from build123d import *

# Parameters (mm, degrees)
SKETCH1_W            = 164
SKETCH1_H            = 264
BOSS_EXTRUDE1_DEPTH  = 4
CUT_EXTRUDE3_DEPTH   = 10
CUT_EXTRUDE4_DEPTH   = 10
LPATTERN1_COUNT      = 3
LPATTERN1_PITCH      = 10
LPATTERN1_COUNT_DIR2 = 2
LPATTERN1_PITCH_DIR2 = 50
CUT_EXTRUDE5_DEPTH   = 10
SKETCH5_W            = 4.319122357
SKETCH5_H            = 26.937684175
SKETCH5_H_2          = 25.730682063
BOSS_EXTRUDE2_DEPTH  = 4
FILLET3_R            = 5
FILLET4_R            = 5
FILLET5_R            = 4.5
FILLET6_R            = 4.5
FILLET7_R            = 4.75
FILLET8_R            = 4.75
FILLET9_R            = 4.5
FILLET10_R           = 4.5


with BuildPart() as part:
    # Sketch1 → Boss-Extrude1 (new body)
    with BuildSketch(Plane.XY):
        with Locations((12.541176471, -29.098039216)):
            Rectangle(SKETCH1_W, SKETCH1_H)
    extrude(amount=BOSS_EXTRUDE1_DEPTH)

    # Sketch2 → Cut-Extrude3 (cut)
    with BuildSketch(Plane.XY.offset(4)):
        with BuildLine():
            ThreePointArc((-19.196819428, 52.401960784), (13.041176471, 20.163964886), (45.279172369, 52.401960784))
            ThreePointArc((45.279172369, 52.401960784), (40.932647519, 56.748485634), (36.58612267, 52.401960784))
            ThreePointArc((36.58612267, 52.401960784), (13.041176471, 28.857014585), (-10.503769729, 52.401960784))
            ThreePointArc((-10.503769729, 52.401960784), (-14.850294578, 56.748485634), (-19.196819428, 52.401960784))
        make_face()
        with BuildLine():
            ThreePointArc((33.426584493, 52.401960784), (13.041176471, 72.787368807), (-7.344231552, 52.401960784))
            ThreePointArc((-7.344231552, 52.401960784), (-2.891363068, 47.949092301), (1.561505415, 52.401960784))
            ThreePointArc((1.561505415, 52.401960784), (13.041176471, 63.88163184), (24.520847526, 52.401960784))
            ThreePointArc((24.520847526, 52.401960784), (28.97371601, 47.949092301), (33.426584493, 52.401960784))
        make_face()
        with BuildLine():
            ThreePointArc((42.181568033, 67.499048907), (12.784631297, 85.219923468), (-16.331673874, 67.04163813))
            ThreePointArc((-16.331673874, 67.04163813), (-14.055015917, 60.240559274), (-7.253937061, 62.517217231))
            ThreePointArc((-7.253937061, 62.517217231), (12.863917084, 75.077467953), (33.17567306, 62.833264313))
            ThreePointArc((33.17567306, 62.833264313), (40.011512844, 60.663209124), (42.181568033, 67.499048907))
        make_face()
        with BuildLine():
            ThreePointArc((-3.609454357, 38.710399181), (12.244809645, 30.859719351), (28.635450382, 37.518379654))
            ThreePointArc((28.635450382, 37.518379654), (28.481389363, 44.125242049), (21.874526968, 43.97118103))
            ThreePointArc((21.874526968, 43.97118103), (12.590075808, 40.199393986), (3.609454357, 44.646398506))
            ThreePointArc((3.609454357, 44.646398506), (-2.967999663, 45.2878532), (-3.609454357, 38.710399181))
        make_face()
    extrude(amount=-CUT_EXTRUDE3_DEPTH, mode=Mode.SUBTRACT)

    # Sketch3 → Cut-Extrude4 (cut)
    with BuildSketch(Plane.XY.offset(4)):
        with BuildLine():
            Line((76.541176471, -57.098039216), (46.541176471, -57.098039216))
            ThreePointArc((46.541176471, -57.098039216), (44.541176471, -55.098039216), (46.541176471, -53.098039216))
            Line((46.541176471, -53.098039216), (76.541176471, -53.098039216))
            ThreePointArc((76.541176471, -53.098039216), (78.541176471, -55.098039216), (76.541176471, -57.098039216))
        make_face()
    cut_extrude4 = extrude(amount=-CUT_EXTRUDE4_DEPTH, mode=Mode.SUBTRACT)

    # LPattern1: Cut-Extrude4 3 × 2
    with Locations(*[(-j * LPATTERN1_PITCH_DIR2, -i * LPATTERN1_PITCH, 0) for i in range(LPATTERN1_COUNT) for j in range(LPATTERN1_COUNT_DIR2) if (i, j) != (0, 0)]):
        add(cut_extrude4, mode=Mode.SUBTRACT)

    # Sketch4 → Cut-Extrude5 (cut)
    with BuildSketch(Plane.XY.offset(4)):
        with BuildLine():
            Line((7.541176471, -143.598039216), (17.541176471, -143.598039216))
            ThreePointArc((17.541176471, -143.598039216), (20.041176471, -146.098039216), (17.541176471, -148.598039216))
            Line((17.541176471, -148.598039216), (7.541176471, -148.598039216))
            ThreePointArc((7.541176471, -148.598039216), (5.041176471, -146.098039216), (7.541176471, -143.598039216))
        make_face()
    extrude(amount=-CUT_EXTRUDE5_DEPTH, mode=Mode.SUBTRACT)

    # Sketch5 → Boss-Extrude2 (add)
    with BuildSketch(Plane.XY.offset(4)):
        with Locations((13.038358708, 73.546081582)):
            Rectangle(SKETCH5_W, SKETCH5_H)
        with Locations((13.038358708, 29.708086806)):
            Rectangle(SKETCH5_W, SKETCH5_H_2)
    extrude(amount=-BOSS_EXTRUDE2_DEPTH)

    # Fillet3
    fillet3_edges = [part.edges().sort_by_distance(p)[0] for p in [
        (15.197919886, 74.975363365, 2),
        (15.197919886, 85.149982831, 2),
    ]]
    fillet(fillet3_edges, radius=FILLET3_R)

    # Fillet4
    fillet4_edges = [part.edges().sort_by_distance(p)[0] for p in [
        (10.878797529, 74.974824217, 2),
        (10.878797529, 85.149611196, 2),
    ]]
    fillet(fillet4_edges, radius=FILLET4_R)

    # Fillet5
    # the kernel refuses this fillet: 4.5 mm, written as the material it adds along each edge
    with BuildSketch(Plane(origin=(10.878797529, 63.676133253, 0), x_dir=(-0.952400444463688, -0.3048497882324502, 0), z_dir=(0, 0, 1))) as fillet5_piece_1:
        with BuildLine():
            CenterArc((3.294924666, -4.467486403), FILLET5_R, 96.891689821, 65.359183141)
            Line((-0.990877334, -3.095662356), (0, 0))
            ThreePointArc((0, 0), (1.377478425, -0.082943423), (2.75495685, 0))
        make_face()
    extrude(amount=4)
    with BuildSketch(Plane(origin=(10.878797529, 72.672357366, 0), x_dir=(0, -1, 0), z_dir=(0, 0, 1))) as fillet5_piece_2:
        with BuildLine():
            CenterArc((5.849616613, -4.5), FILLET5_R, 90, 114.796867003)
            ThreePointArc((1.764514753, -6.387310996), (0.620984955, -3.265832826), (0, 0))
            Line((0, 0), (5.849616613, 0))
        make_face()
    extrude(amount=4)

    # Fillet6
    # the kernel refuses this fillet: 4.5 mm, written as the material it adds along each edge
    with BuildSketch(Plane(origin=(15.197919886, 72.672957753, 0), x_dir=(0.963984906204346, -0.2659569525509686, 0), z_dir=(0, 0, 1))) as fillet6_piece_1:
        with BuildLine():
            CenterArc((5.893145872, -4.440206052), FILLET6_R, 80.649344531, 114.774478291)
            Line((1.555213794, -5.637012339), (0, 0))
            ThreePointArc((0, 0), (3.312144479, 0.270872005), (6.624288959, 0))
        make_face()
    extrude(amount=4)
    with BuildSketch(Plane(origin=(15.197919886, 63.677212683, 0), x_dir=(0.9525356739175572, -0.30442698617965064, 0), z_dir=(0, 0, 1))) as fillet6_piece_2:
        with BuildLine():
            CenterArc((3.296449531, 4.467456192), FILLET6_R, 197.723693353, 65.381411924)
            Line((-0.989961002, 3.097534754), (0, 0))
            ThreePointArc((0, 0), (1.378115911, 0.083020491), (2.756231822, 0))
        make_face()
    extrude(amount=4)

    # Fillet7
    # the kernel refuses this fillet: 4.75 mm, written as the material it adds along each edge
    with BuildSketch(Plane(origin=(15.197919886, 30.953165389, 0), x_dir=(0, 1, 0), z_dir=(0, 0, 1))) as fillet7_piece_1:
        with BuildLine():
            CenterArc((6.126567217, -4.75), FILLET7_R, 90, 114.26424477)
            ThreePointArc((1.796182676, -6.701991222), (0.626677135, -3.423736603), (0, 0))
            Line((0, 0), (6.126567217, 0))
        make_face()
    extrude(amount=4)
    with BuildSketch(Plane(origin=(15.197919886, 40.383034621, 0), x_dir=(0.9557846908185708, 0.2940673813887714, 0), z_dir=(0, 0, 1))) as fillet7_piece_2:
        with BuildLine():
            CenterArc((3.51897249, -4.715313748), FILLET7_R, 96.928419065, 65.969959025)
            Line((-1.021004791, -3.318493687), (0, 0))
            ThreePointArc((0, 0), (1.472991805, -0.08916851), (2.94598361, 0))
        make_face()
    extrude(amount=4)

    # Fillet8
    # the kernel refuses this fillet: 4.75 mm, written as the material it adds along each edge
    with BuildSketch(Plane(origin=(10.878797529, 40.384047255, 0), x_dir=(0, -1, 0), z_dir=(0, 0, 1))) as fillet8_piece_1:
        with BuildLine():
            CenterArc((3.470508434, -4.75), FILLET8_R, 90, 65.949113414)
            ThreePointArc((-0.867114896, -2.814147772), (-0.348416422, -1.433308135), (0, 0))
            Line((0, 0), (3.470508434, 0))
        make_face()
    extrude(amount=4)
    with BuildSketch(Plane(origin=(10.878797529, 30.953732806, 0), x_dir=(-0.9658301221176608, 0.2591759541511984, 0), z_dir=(0, 0, 1))) as fillet8_piece_2:
        with BuildLine():
            CenterArc((6.176063632, -4.688044059), FILLET8_R, 80.735851864, 114.285319943)
            Line((1.588370552, -5.919129841), (0, 0))
            ThreePointArc((0, 0), (3.470374234, 0.281175054), (6.940748468, 0))
        make_face()
    extrude(amount=4)

    # Fillet9
    # the kernel refuses this fillet: 4.5 mm, written as the material it adds along each edge
    with BuildSketch(Plane(origin=(10.878797529, 20.23656794, 0), x_dir=(0, 1, 0), z_dir=(0, 0, 1))) as fillet9_piece_1:
        with BuildLine():
            CenterArc((5.239399394, 4.5), FILLET9_R, 166.10226732, 103.89773268)
            ThreePointArc((0.871132452, 5.58085333), (0.313102845, 2.809542348), (0, 0))
            Line((0, 0), (5.239399394, 0))
        make_face()
    extrude(amount=4)
    with BuildSketch(Plane(origin=(10.878797529, 28.956521807, 0), x_dir=(-0.9862681446857605, 0.16515189002281502, 0), z_dir=(0, 0, 1))) as fillet9_piece_2:
        with BuildLine():
            CenterArc((3.811181811, 4.487703929), FILLET9_R, 189.50605818, 76.257380527)
            Line((-0.62702484, 3.744520424), (0, 0))
            ThreePointArc((0, 0), (1.739373093, 0.064335629), (3.478746186, 0))
        make_face()
    extrude(amount=4)

    # Fillet10
    # the kernel refuses this fillet: 4.5 mm, written as the material it adds along each edge
    with BuildSketch(Plane(origin=(15.197919886, 20.236189577, 0), x_dir=(0.9880653050237032, 0.15403555761062557, 0), z_dir=(0, 0, 1))) as fillet10_piece_1:
        with BuildLine():
            CenterArc((5.253191268, 4.482705444), FILLET10_R, 171.139133949, 103.885741164)
            Line((0.806897395, 5.175865453), (0, 0))
            ThreePointArc((0, 0), (2.823669163, -0.123898184), (5.647338326, 0))
        make_face()
    extrude(amount=4)
    with BuildSketch(Plane(origin=(15.197919886, 28.956002724, 0), x_dir=(0.9863050503076972, 0.16493134249599425, 0), z_dir=(0, 0, 1))) as fillet10_piece_2:
        with BuildLine():
            CenterArc((3.812043631, -4.48769836), FILLET10_R, 94.237521054, 76.269232907)
            Line((-0.626329096, -3.745507319), (0, 0))
            ThreePointArc((0, 0), (1.739766416, -0.064364768), (3.479532832, 0))
        make_face()
    extrude(amount=4)


solid = part.part
Here's how the part is built. I have some questions about the finished solid (model axes, mm). A direction names the side the tool comes from. Give positions to 0.01 mm unless a question says otherwise; leave off trailing zeros. Loops run counter-clockwise (first coordinate to the right, second up) from the corner with the lowest first, then second, coordinate; pieces in that order, holes last. Notation, with made-up numbers: (57, 19) -> (116, 19) arc R19 ccw to (116, 29) -> close; hole circle Ø11 at (72, -37.75). An arc over 180 degrees is marked (long way). Answer as a JSON object with one key per item and string values. Group by question number.
Item 1: Imagine slicing it at B-B on z = 2.55. Give the number of separate pieces and of enclosed holes in the cut face, then the cut area to 3 significant figures.
Item 2: On a 3-axis mill with a long thin cutter (end or side, diameter ignored), from which of +Z, -Z, +X, -X, +Y, -Y can I reach the whole of each face in a straight line? I mean faces 3 (the flat face through (14, -27, 0)), 4 (the cylindrical face through (3.33, 58.52, 2.03)). Say none if no direction works.
Item 3: Imagine slicing it at A-A on x = 54. Write out the boundary of the cut face in (y, z).
Item 4: Thinking about a two-plate mould opening in X: for faces 1 (the cylindrical face through (31.7, 38.04, 2.03)), 2 (the flat face through (14, -27, 4)), which applies, pulls with the +X half, pulls with the -X half, needs draft (parallel to the pull), parting line crosses it, or undercut?
Item 5: I need wall thicknesses on L1, parallel to X at y = -75.5, z = 2.4; L2, parallel to X at y = 36.5, z = 2.6; L3, parallel to Y at x = 29.5, z = 2.6. Which ranges of each line are inside material? Lowest first, please.
Item 6: Will this pin go through, and if not, where does the flat tip stop? pin 1 (5 mm diameter, centred on x = 3, y = -50, fed in from -Z).
Answer list:
{
 "1": {"separate pieces": "1", "enclosed holes": "15", "area": "40,300 mm2"},
 "2": {"face 3": "-Z, +X, -X, +Y, -Y", "face 4": "+Z, -Z"},
 "3": {"outline": "(-161.1, 0) -> (-77.1, 0) -> (-77.1, 4) -> (-161.1, 4) -> close; (-73.1, 0) -> (-67.1, 0) -> (-67.1, 4) -> (-73.1, 4) -> close; (-63.1, 0) -> (-57.1, 0) -> (-57.1, 4) -> (-63.1, 4) -> close; (-53.1, 0) -> (102.9, 0) -> (102.9, 4) -> (-53.1, 4) -> close"},
 "4": {"face 1": "undercut", "face 2": "needs draft"},
 "5": {"L1": "x = -69.46 to -5.42, 28.5 to 44.58, 78.5 to 94.54", "L2": "x = -69.46 to -15, -4.32 to -1.51, 10.84 to 15.23, 27.6 to 30.4, 41.08 to 94.54", "L3": "y = -161.1 to 24.68, 35.57 to 38.79, 42.7 to 47.98, 64.43 to 68, 80.8 to 102.9"},
 "6": {"pin 1": "stops at z = 0"}
}
